Autodesk Inventor part; units mm, degrees
ref_plane "YZ Plane" through (0, 0, 0) normal (1, 0, 0) x (0, 1, 0)
ref_plane "XZ Plane" through (0, 0, 0) normal (0, 1, 0) x (-1, 0, 0)
ref_plane "XY Plane" through (0, 0, 0) normal (0, 0, 1) x (1, 0, 0)
sketch "Esboço1" plane through (0, 0, 0) normal (0, 0, 1) x (1, 0, 0)
  line L0 (-20, -40) -> (20, -40)
  line L1 (20, -40) -> (20, 40)
  line L2 (20, 40) -> (-20, 40)
  line L3 (-20, 40) -> (-20, -40)
  line L4 (-20, 40) -> (20, 40)
  circle A0 centre (0, 30) radius 5 construction
  circle A1 centre (0, 30) radius 28 construction
  circle A2 centre (0, 30) radius 74 construction
  line L5 (-20, 10.4041) -> (20, 10.4041) construction
  line L6 (-20, -44) -> (20, -44) construction
  line L7 (-103.6, 0) -> (103.6, 0) construction
  line L8 (0, -73.6) -> (0, 133.6) construction
  line L9 (-20, 16.906) -> (20, 40)
  point P0 (0, 0)
  dimension "d0" = 80
  dimension "d1" = 40
  dimension "d41" = 10
  dimension "d42" = 70
  dimension "d43" = 56
  dimension "d45" = 84
  dimension "d49" = 30
  dimension "d58" = 10
extrude "Extrusão1" add sketch "Esboço1" along normal mid plane 10
extrude "Extrusão4" [suppressed]
sketch "Esboço2" plane through (-20, -40, -5) normal (0, -1, 0) x (1, 0, 0)
  line L0 (40, 10) -> (40, 0)
  line L1 (40, 5) -> (0, 5) construction
  line L2 (0, 0) -> (0, 10)
  line L3 (0, 0) -> (0, 10)
  line L4 (40, 0) -> (40, 10)
  line L5 (0, 10) -> (40, 10) construction
  line L6 (20, 10) -> (20, 0) construction
  line L7 (40, 0) -> (0, 0) construction
  point P0 (20, 5)
  point P1 (7.5, 5)
  point P2 (32.5, 5)
  dimension "d9" = 7.5
  dimension "d10" = 7.5
  dimension "d37" = 25
hole "Furo1" at (-12.5, -40, 0) at (12.5, -40, 0) direction (0, 1, 0) diameter 3.242 depth 15 tip angle 118
sketch "Esboço3" plane through (0, 0, 5) normal (0, 0, 1) x (1, 0, 0)
  point P0 (0, 0)
  point P1 (0, 37.5)
  point P2 (0, 30)
hole "Furo2" [suppressed]
sketch "Esboço6" plane through (20, 40, 5) normal (-0.5, 0.8660254, 0) x (0.8660254, 0.5, 0)
  line L0 (0, 0) -> (0, 10) construction
  line L1 (0, 5) -> (-46.188, 5) construction
  line L2 (-46.188, 0) -> (-46.188, 10) construction
  line L3 (-23.094, 5) -> (-23.094, 0) construction
  point P0 (-37.3205, 5)
  point P1 (-33.094, 5)
  point P2 (-13.094, 5)
  dimension "d50" = 20
hole "Furo3" [suppressed]
sketch "Esboço7" plane through (-20, 40, 5) normal (0, 1, 0) x (1, 0, 0)
  line L0 (-8, 5) -> (48, 5) construction
  line L1 (20, 12) -> (20, -2) construction
  line L2 (0, 10) -> (0, 0)
  point P0 (20, 5)
  point P1 (14.86, 5)
  dimension "d59" = 14.86
hole "Furo4" at (-5.14, 40, 0) direction (0, -1, 0) diameter 3.242 depth 15 tip angle 118 countersink diameter 10 countersink angle 90
fillet "Arredondamento3" radius 2 2 edges at (20, 40, 0) (-20, 40, 0)
properties part number "GRJ-03-116B" material "Fenolite OR"
Here's how the part is built. I have some questions about the finished solid (model axes, mm). A direction names the side the tool comes from. Round coordinates to 2 decimals unless told otherwise and drop trailing zeros. One line per question, with ' | ' between items. Start each with the question number.
Q1. We'd pull the mould along X, two halves only. Please class faces 1 (the flat face through (20, -2, 0)), 2 (the flat face through (0, -40, 0)), 3 (the cylindrical face through (10.893, -32.395, 0.211)): +X half, -X half, draft (parallel to the pull), parting line (faces both ways), or undercut.
Q2. Will this pin go through, and if not, where does the flat tip stop? pin 1 (1.9 mm diameter, centred on x = -12.5, z = 0, fed in from -Y).
Q3. Please list where these lines run through material, in increasing order: line 1 (X direction, y = -35.5, z = 0); line 2 (Z direction, x = 12.5, y = -31.5); line 3 (X direction, y = 29.75, z = 0). Write a range as [from, to].
Q4. For faces 4 (the flat face through (-13, 40, 0)), 5 (the cylindrical face through (-14.107, -32.395, 0.211)), 6 (the cylindrical face through (-3.702, 30.729, 0.748)), which set-ups out of +Z, -Z, +X, -X, +Y, -Y let a thin tool reach every point of the face, with its end or its side?
Response values:
1) face 1: +X half | face 2: draft | face 3: undercut
2) pin 1: stops at y = -24.6
3) line 1: x = [-20, -14.12], [-10.88, 10.88], [14.12, 20] | line 2: z = [-5, -1.62], [1.62, 5] | line 3: x = [-20, -6.76], [-3.52, 20]
4) face 4: +Z, -Z, +X, -X, +Y | face 5: -Y | face 6: +Y
